Autodesk Inventor part; units mm, degrees
ref_plane "YZ Plane" through (0, 0, 0) normal (1, 0, 0) x (0, 1, 0)
ref_plane "XZ Plane" through (0, 0, 0) normal (0, 1, 0) x (-1, 0, 0)
ref_plane "XY Plane" through (0, 0, 0) normal (0, 0, 1) x (1, 0, 0)
sketch "Esboço1" plane through (0, 0, 0) normal (0, 1, 0) x (-1, 0, 0)
  line L0 (12, 23) -> (-12, 23)
  line L1 (-12, 23) -> (-12, -23)
  line L2 (-12, -23) -> (12, -23)
  line L3 (12, -23) -> (12, 23)
  line L4 (12, 23) -> (-12, -23) construction
  line L5 (-12, 23) -> (12, -23) construction
  point P0 (0, 0)
  dimension "d0" = 24
  dimension "d1" = 46
extrude "Base" add sketch "Esboço1" along normal blind 3
sketch "Esboço2" plane through (0, 3, 0) normal (0, 1, 0) x (1, 0, 0)
  line L0 (-9.5, -20.5) -> (9.5, -20.5)
  line L1 (9.5, -20.5) -> (9.5, 20.5)
  line L2 (9.5, 20.5) -> (-9.5, 20.5)
  line L3 (-9.5, 20.5) -> (-9.5, -20.5)
  line L4 (-9.5, -20.5) -> (9.5, 20.5) construction
  line L5 (9.5, -20.5) -> (-9.5, 20.5) construction
  line L6 (-12, 23) -> (-12, -23)
  point P0 (0, 0)
  dimension "d4" = 19
  dimension "d5" = 41
extrude "Encaixe" add sketch "Esboço2" along normal blind 2
sketch "Esboço3" plane through (0, 0, 0) normal (0, -1, 0) x (1, 0, 0)
  circle A0 centre (0, 0) radius 6.5
  circle A1 centre (0, 0) radius 5
  dimension "d9" = 13
  dimension "d10" = 10
extrude "Furo" cut sketch "Esboço3" against normal up to surface (5 mm away) contours A1
extrude "Haste" add sketch "Esboço3" along normal blind 60
ref_plane "Plano de trabalho1" through (0, 0, -23) normal (-1, 0, 0) x (0, 0, 1)
sketch "Esboço5" plane through (0, 0, -23) normal (-1, 0, 0) x (0, 0, 1)
  line L0 (17.4096, -19.7038) -> (17.4096, 1.7927)
  line L1 (46, 0) -> (0, 0)
  line L2 (28, -60) -> (28, 5)
  arc A0 (17.4096, -19.7038) -> (11, 0) centre (2.6099, -13.6237) ccw
  line L3 (23, -21.6532) -> (23, 7.4929)
  line L4 (0, 0) -> (46, 0)
  point P0 (23, 0)
  point P1 (26.9955, 0)
  point P2 (23, 0)
  point P3 (23, 0)
  point P4 (17.4096, -7.5437)
  point P5 (17.4096, 0)
  dimension "d25" = 16
  dimension "d27" = 12
revolve "Revolução1" add sketch "Esboço5" angle 360 about axis through (0, -21.6532, 0) along (0, 1, 0) contours A0 L1 L0
properties part number "Tampa Eletroimã"
Can you work these out from the model? Positions are in its coordinate system, mm. A direction names the side the tool comes from. Round coordinates to 2 decimals unless told otherwise and drop trailing zeros. Loops run counter-clockwise (first coordinate to the right, second up) from the corner with the lowest first, then second, coordinate; pieces in that order, holes last. Notation, with made-up numbers: M 83,-4.5 L 111,-4.5 A30 cw 111,26.5 Z; hole C -23.5,58.25 d2. An arc over 180 degrees is marked long. Answer in a Markdown table with one row per item.
1. I'm going to push flat-ended pins straight in: pin 1 Ø7 at (x, z) = (3.5, 13) entering from -Y; pin 2 Ø0.6 at (x, y) = (-2.5, 3.5) entering from -Z; pin 3 Ø12 at (x, z) = (-5.5, 17) entering from -Y; pin 4 Ø11.5 at (x, z) = (0, 0) entering from -Y. Where does each tip first touch, or does it pass through?
Established:
| item | result |
|---|---|
| pin 1 | y = -1.49 |
| pin 2 | z = -20.5 |
| pin 3 | y = -0.08 |
| pin 4 | y = -60 |
2. Please list where these lines run through material, in increasing order: line 1 (Z direction, x = 0.25, y = -18.5); line 2 (Y direction, x = 3, z = -19.5); line 3 (Y direction, x = -10, z = 20). Write a range as from..to.
Established:
| item | result |
|---|---|
| line 1 | -6.5..-4.99, 4.99..6.5 |
| line 2 | 0..5 |
| line 3 | 0..3 |
3. If we section it at B-B, the plane z = 16: Please give me the cut outline in (x, y).
Established:
| item | result |
|---|---|
| outline | M -12,0 L 12,0 L 12,3 L 9.5,3 L 9.5,5 L -9.5,5 L -9.5,3 L -12,3 Z |
4. Thinking about a two-plate mould opening in Z: for faces 1 (the face through (-1.08, -27.04, 4.88)), 2 (the face through (2, -60, -5)), 3 (the face through (-5.158, -32.461, 3.955)), which applies, pulls with the +Z half, pulls with the -Z half, needs draft (parallel to the pull), parting line crosses it, or undercut?
Established:
| item | result |
|---|---|
| face 1 | undercut |
| face 2 | needs draft |
| face 3 | parting line crosses it |
5. If we section it at A-A, the plane x = 0: Please give me the cut outline in (y, z).
Established:
| item | result |
|---|---|
| outline | M -60,-6.5 L -5.68,-6.5 A16 cw 0,-12 L 0,-23 L 3,-23 L 3,-20.5 L 5,-20.5 L 5,-5 L -60,-5 Z; M -60,5 L 5,5 L 5,20.5 L 3,20.5 L 3,23 L 0,23 L 0,12 A16 cw -5.68,6.5 L -60,6.5 Z |
6. If we section it at C-C, the plane y = -22: Please give me the cut outline in (x, z).
Established:
| item | result |
|---|---|
| outline | C 0,0 d13; hole C 0,0 d10 |
7. On a 3-axis mill with a long thin cutter (end or side, diameter ignored), from which of +Z, -Z, +X, -X, +Y, -Y can I reach the whole of each face in a straight line? I mean faces 4 (the face through (9.5, 4, 0)), 5 (the face through (-9.5, 4, 0)), 6 (the face through (0, 4, -20.5)). Say none if no direction works.
Established:
| item | result |
|---|---|
| face 4 | +Z, -Z, +X, +Y |
| face 5 | +Z, -Z, -X, +Y |
| face 6 | -Z, +X, -X, +Y |
